```python
from build123d import *

# Parameters (mm, degrees)
SKETCH_R     = 1.5
PAD_DEPTH    = 6
SKETCH001_R  = 1.25
PAD001_DEPTH = 6
CHAMFER_SIZE = 0.25


with BuildPart() as part:
    # Sketch → Pad (new body)
    with BuildSketch(Plane.XY):
        Circle(SKETCH_R)
    extrude(amount=PAD_DEPTH)

    # Sketch001 (on Face3 of Pad) → Pad001 (join)
    with BuildSketch(Plane.XY.offset(6)):
        Polygon((0, -3.290897), (2.85, -1.645448), (2.85, 1.645448), (0, 3.290897), (-2.85, 1.645448), (-2.85, -1.645448), align=None)
        Circle(SKETCH001_R, mode=Mode.SUBTRACT)
    extrude(amount=PAD001_DEPTH)

    # Chamfer
    chamfer_edges = [part.edges().sort_by_distance(p)[0] for p in [
        (-1.5, 0, 0),
    ]]
    chamfer(chamfer_edges, length=CHAMFER_SIZE)


solid = part.part
```
Work out the finished part from the listing and answer in its coordinate system (mm). A direction names the side the tool comes from. Coordinates: 2 decimals unless noted, no trailing zeros. Write each loop counter-clockwise with the first axis right and the second up, starting at its lowest first coordinate (ties: lowest second). Pieces come first, ordered by that corner, then holes.
Q1. A cutting plane is placed at A-A, the plane z = 6.25. Give the vertices of the cut face in (x, y).
Q2. A cutting plane is placed at B-B, the plane y = 0. Give the vertices of the cut face in (x, z), then the cut area to 3 significant figures.
Q3. Each of these flat-tipped pins is pushed along its axis until it touches: pin 1 Ø0.8 at (x, y) = (-0.5, 0.5) entering from +Z; pin 2 Ø2 at (x, z) = (-1.5, 6) entering from -Y. Where does it stop, or does it pass through?
Q4. A cutting plane is placed at D-D, the plane x = 2.4. Give the vertices of the cut face in (y, z).
Q5. Find the intervals of material crossed by line 1 (X direction, y = 0.75, z = 9.5); line 2 (Y direction, x = -0.4, z = 7.75); line 3 (Z direction, x = -0.1, y = -0.75), in increasing order.
Q6. Determine the mould class of faces 1 (the face through (0, 0, 6)), 2 (the face through (-2.85, 0, 9)), 3 (the face through (2.85, 0, 9)) for opening direction X: released by +X, released by -X, zero draft, split by the parting line, or undercut.
Q7. Which of the six approach directions +Z, -Z, +X, -X, +Y, -Y give full straight-line access (tool end or side, diameter ignored) to faces 4 (the face through (-1.5, 0.07, 3.08)), 5 (the face through (1.405, -2.48, 8.958)), 6 (the face through (-0.27, -1.22, 8.96))?
Q8. A cutting plane is placed at C-C, the plane z = 2.5. Give the vertices of the cut face in (x, y).
Findings below:
1. outline: (-2.85, -1.65) - (0, -3.29) - (2.85, -1.65) - (2.85, 1.65) - (0, 3.29) - (-2.85, 1.65) - close; hole circle Ø2.5 at (0, 0)
2. outline: (-2.85, 6) - (-1.5, 6) - (-1.5, 0.25) - (-1.25, 0) - (1.25, 0) - (1.5, 0.25) - (1.5, 6) - (2.85, 6) - (2.85, 12) - (1.25, 12) - (1.25, 6) - (-1.25, 6) - (-1.25, 12) - (-2.85, 12) - close
2. area: 37.1 mm2
3. pin 1: stops at z = 6
3. pin 2: stops at y = -3
4. outline: (-1.91, 6) - (1.91, 6) - (1.91, 12) - (-1.91, 12) - close
5. line 1: x = -2.85 to -1, 1 to 2.85
5. line 2: y = -3.06 to -1.18, 1.18 to 3.06
5. line 3: z = 0 to 6
6. face 1: undercut
6. face 2: released by -X
6. face 3: released by +X
7. face 4: -Z
7. face 5: +Z, -Z, +X, -Y
7. face 6: +Z
8. outline: circle Ø3 at (0, 0)
